Check sheet for the modelled part. Datum: model origin and axes. Units: mm. A direction names the side the tool comes from. Give positions to 0.01 mm unless a question says otherwise; leave off trailing zeros. Write each loop counter-clockwise with the first axis right and the second up, starting at its lowest first coordinate (ties: lowest second). Pieces come first, ordered by that corner, then holes. Notation, with made-up numbers: M -19,22.5 L 27,22.5 A23 cw 27,36.5 Z; hole C 68,22 d10. An arc over 180 degrees is marked long. Write item = value, one per line. Start each with the question number.
1) Gauge pin test, flat ends, axial feed: pin 1 (4 mm diameter, centred on x = 2.5, z = -2, fed in from +Y); pin 2 (5 mm diameter, centred on y = 4.5, z = -10.5, fed in from -X); pin 3 (6 mm diameter, centred on x = 17.5, y = 9.5, fed in from +Z); pin 4 (18 mm diameter, centred on x = -48, z = 0, fed in from -Y). Record the tip position at first contact, or that the pin passes through.
2) Draft check along X on faces 3 (the face through (-35.35, 12.46, 8.06)), 4 (the face through (37, 5, 20)), 5 (the face through (-57.76, 7.4, -2.17)). Enter one of: pulls with the +X half, pulls with the -X half, needs draft (parallel to the pull), parting line crosses it, or undercut.
3) Sectioned sample at A-A, the plane x = 0. Record the cut outline in (y, z), then the cut area to 3 significant figures.
4) Sectioned sample at B-B, the plane z = 0. Record the cut outline in (x, y), then the cut area to 3 significant figures.
5) Set-up check for faces 1 (the face through (38.24, 4.93, -2.17)), 2 (the face through (37, 5, -20)): record each of +Z, -Z, +X, -X, +Y, -Y from which the full face is reachable in a straight line by a thin tool's end or side.
6) Scan lines: L1, parallel to X at y = 5.75, z = 0; L2, parallel to Y at x = 6, z = -12; L3, parallel to X at y = 6, z = 26.5. Record each from-to range of solid material in increasing order.
7) Sectioned sample at C-C, the plane y = 12.5. Record the cut outline in (x, z), then the cut area to 3 significant figures.
8) Sectioned sample at D-D, the plane x = -60. Record the cut outline in (y, z).
from build123d import *

# Parameters (mm, degrees)
SKETCH1_R           = 5
SKETCH1_R_2         = 10
BOSS_EXTRUDE1_DEPTH = 10
SKETCH2_R           = 15
SKETCH2_R_2         = 10
BOSS_EXTRUDE2_DEPTH = 5


with BuildPart() as part:
    # Sketch1 → Boss-Extrude1 (new body)
    with BuildSketch(Plane(origin=(0, 0, 0), x_dir=(1, 0, 0), z_dir=(0, 1, 0))):
        with BuildLine():
            Line((12, 30), (-48, 30))
            ThreePointArc((-48, 30), (-78, 0), (-48, -30))
            Line((-48, -30), (12, -30))
            ThreePointArc((12, -30), (17.481881586, -22.752551286), (26.142135624, -20))
            Line((26.142135624, -20), (48, -20))
            ThreePointArc((48, -20), (68, 0), (48, 20))
            Line((48, 20), (26.142135624, 20))
            ThreePointArc((26.142135624, 20), (17.481881586, 22.752551286), (12, 30))
        make_face()
        with Locations(Location((0, 0, 0), (0, 0, 270))):  # turned: the seam where the file's is
            Circle(SKETCH1_R, mode=Mode.SUBTRACT)
        with Locations(Location((-48, 0, 0), (0, 0, 270))):  # turned: the seam where the file's is
            Circle(SKETCH1_R_2, mode=Mode.SUBTRACT)
        with Locations(Location((48, 0, 0), (0, 0, 270))):  # turned: the seam where the file's is
            Circle(SKETCH1_R_2, mode=Mode.SUBTRACT)
    extrude(amount=BOSS_EXTRUDE1_DEPTH)

    # Sketch2 → Boss-Extrude2 (add)
    with BuildSketch(Plane(origin=(0, 10, 0), x_dir=(1, 0, 0), z_dir=(0, 1, 0))):
        with Locations(Location((-48, 0, 0), (0, 0, 270))):  # turned: the seam where the file's is
            Circle(SKETCH2_R)
        with Locations(Location((-48, 0, 0), (0, 0, 270))):  # turned: the seam where the file's is
            Circle(SKETCH2_R_2, mode=Mode.SUBTRACT)
    extrude(amount=BOSS_EXTRUDE2_DEPTH)


solid = part.part
Data:
q1.pin_1 = 10
q1.pin_2 = -76.91
q1.pin_3 = 25.54
q1.pin_4 = through
q2.face_3 = parting line crosses it
q2.face_4 = needs draft
q2.face_5 = undercut
q3.outline = M 0,-30 L 10,-30 L 10,-5 L 0,-5 Z; M 0,5 L 10,5 L 10,30 L 0,30 Z
q3.area = 500 mm2
q4.outline = M -78,0 L -58,0 L -58,15 L -63,15 L -63,10 L -78,10 Z; M -38,0 L -5,0 L -5,10 L -33,10 L -33,15 L -38,15 Z; M 5,0 L 38,0 L 38,10 L 5,10 Z; M 58,0 L 68,0 L 68,10 L 58,10 Z
q4.area = 1,010 mm2
q5.face_1 = +Y, -Y
q5.face_2 = -Z, +X, +Y, -Y
q6.L1 = -78 to -58, -38 to -5, 5 to 38, 58 to 68
q6.L2 = 0 to 10
q6.L3 = -62.06 to 13.78
q7.outline = C -48,0 d30; hole C -48,0 d20
q7.area = 393 mm2
q8.outline = M 0,-27.5 L 10,-27.5 L 10,-9 L 15,-9 L 15,9 L 10,9 L 10,27.5 L 0,27.5 Z
